Geometry check sheet. Reference: drawing and pictorial views, mm from the part's lowest x, y, z. A direction names the side the tool comes from. Round coordinates to 2 decimals unless told otherwise and drop trailing zeros. Order: outer loops, then holes, each group sorted by start corner. A loop starts at its lowest first (then second) coordinate and runs counter-clockwise, first axis right, second up.
(1) Mould release check, pull along Y, two halves, no side actions. Record for the marked faces 4, 5 and 6: released by +Y, released by -Y, zero draft, split by the parting line, or undercut.
(2) Sectioned sample at C-C, the plane x = 58. Enter the section's corners in (y, z) (3 decimals).
(3) Thickness scan on probe 1 along X at (y, z) = (1.75, 25.4); probe 2 along X at (y, z) = (5.75, 17.5) (3 decimals); probe 3 along Y at (x, z) = (53, 19.5) (3 decimals). Record the ranges inside material, lowest first.
(4) Depth check by flat-ended pin: pin 1 (3.5 mm diameter, centred on x = 13, y = 1.5, fed in from +Z); pin 2 (2.5 mm diameter, centred on x = 11.5, y = 1.5, fed in from -Z); pin 3 (4 mm diameter, centred on y = 9.5, z = 14.5, fed in from +X) (3 decimals). Enter the tip coordinate at first touch or a pass-through.
(5) Sectioned sample at A-A, the plane z = 25.4. Count the separate pieces of the cut face and the enclosed holes in it, and give its area (3 significant figures).
(6) Sectioned sample at D-D, the plane z = 41. Enter the section's corners in (x, y) (3 decimals), and give its area (3 significant figures).
(7) Tool access check on the marked faces 1, 2 and 3. Record the directions out of +Z, -Z, +X, -X, +Y, -Y that give a thin tool (end or side, any length) a straight path to the whole face; none if there is none.
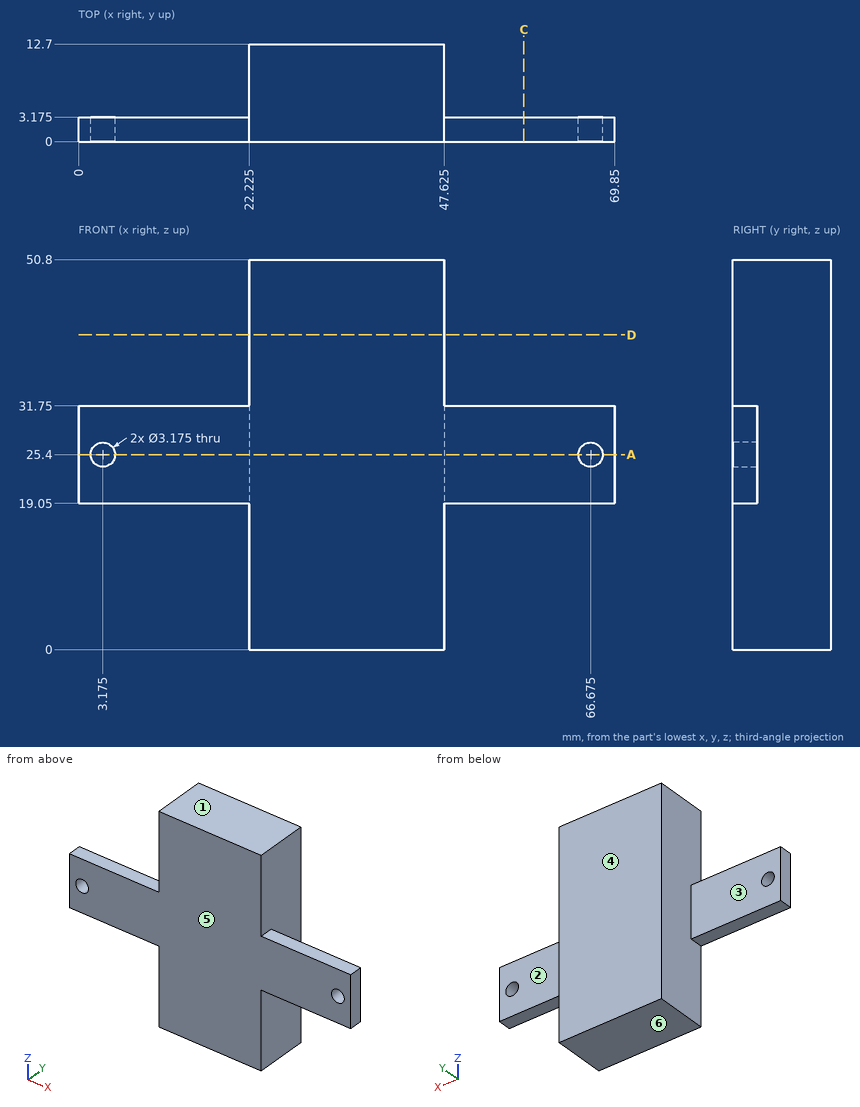
Derived:
1. face 4: released by +Y
1. face 5: released by -Y
1. face 6: zero draft
2. outline: (0, 19.05) - (3.175, 19.05) - (3.175, 31.75) - (0, 31.75) - close
3. probe 1: x = 0 to 1.59, 4.76 to 65.09, 68.26 to 69.85
3. probe 2: x = 22.225 to 47.625
3. probe 3: y = 0 to 3.175
4. pin 1: stops at z = 31.75
4. pin 2: stops at z = 19.05
4. pin 3: stops at x = 47.625
5. separate pieces: 3
5. enclosed holes: 0
5. area: 444 mm2
6. outline: (22.225, 0) - (47.625, 0) - (47.625, 12.7) - (22.225, 12.7) - close
6. area: 323 mm2
7. face 1: +Z, +X, -X, +Y, -Y
7. face 2: +Z, -Z, +X, +Y
7. face 3: +Z, -Z, -X, +Y
